Could you check a few things on this model? Use its own coordinates, in mm. A direction names the side the tool comes from. Round coordinates to 2 decimals unless told otherwise and drop trailing zeros. Order: outer loops, then holes, each group sorted by start corner. A loop starts at its lowest first (then second) coordinate and runs counter-clockwise, first axis right, second up. Notation, with made-up numbers: (50.5, 69) - (71.5, 69) arc R15 ccw to (71.5, 79) - close; hole circle Ø7 at (7.5, -31.5). An arc over 180 degrees is marked (long way). Use one line per item in the form item = value.
from build123d import *

# Parameters (mm, degrees)
F1_DEPTH = 63.5
F0_W     = 18.9613934278
F0_H     = 19.05
F2_DEPTH = 19.05
F3_DEPTH = 7.9375
F5_R     = 6.35


with BuildPart() as f1:
    # F0 (on Front) → F1 (new body, symmetric)
    with BuildSketch(Plane.XZ):
        Polygon((63.5, -19.05), (63.5, 19.05), (44.45, 19.05), (-63.5, 19.05), (-63.5, -19.05), align=None)
    extrude(amount=F1_DEPTH, both=True)

    # F0 (on Front) → F2 (join, symmetric)
    with BuildSketch(Plane.XZ):
        with Locations((98.3806967139, 73.025)):
            Rectangle(F0_W, F0_H)
        with BuildLine():
            Line((44.45, 19.05), (63.5, 19.05))
            Line((63.5, 19.05), (63.5, 50.8))
            ThreePointArc((63.5, 50.8), (67.2197438789, 59.7802561211), (76.2, 63.5))
            Line((76.2, 63.5), (88.9, 63.5))
            Line((88.9, 63.5), (88.9, 82.55))
            Line((88.9, 82.55), (76.2, 82.55))
            ThreePointArc((76.2, 82.55), (53.7493596973, 73.2506403027), (44.45, 50.8))
            Line((44.45, 50.8), (44.45, 19.05))
        make_face()
    extrude(amount=F2_DEPTH, both=True)

    # F0 (on Front) → F3 (join, symmetric)
    with BuildSketch(Plane.XZ):
        with BuildLine():
            Line((-63.5, 19.05), (44.45, 19.05))
            Line((44.45, 19.05), (44.45, 50.8))
            ThreePointArc((44.45, 50.8), (53.7493596973, 73.2506403027), (76.2, 82.55))
            add(Edge.make_bspline(
                [(-63.5, 19.05), (-43.5108728707, 70.1786652207), (14.7244036198, 83.1460282207), (76.2, 82.55)],
                knots=[0, 0, 0, 0, 153.4546838647, 153.4546838647, 153.4546838647, 153.4546838647], degree=3))
        make_face()
    extrude(amount=F3_DEPTH, both=True)

    # F0 (on Front) → F4 (revolve)
    with BuildSketch(Plane.XZ):
        Polygon((107.8613934278, 82.55), (107.8613934278, 63.5), (107.8613934278, 57.15), (127, 57.15), (127, 88.9), (107.8613934278, 88.9), align=None)
    revolve(axis=Axis((107.8613934278, 0, 73.025), (0, 0, 1)))

    # F5
    f5_edges = [f1.edges().sort_by_distance(p)[0] for p in [
        (-63.5, 63.5, 0),
        (-63.5, -63.5, 0),
        (63.5, -63.5, 0),
        (63.5, 63.5, 0),
    ]]
    fillet(f5_edges, radius=F5_R)


solid = f1.part
Item 1: Imagine slicing it at B-B on x = 97. Please give me the cut outline in (y, z), plus the area to 3 significant figures.
Found:
outline = (-19.05, 63.5) - (-15.76, 63.5) - (-15.76, 57.15) - (15.76, 57.15) - (15.76, 63.5) - (19.05, 63.5) - (19.05, 82.55) - (15.76, 82.55) - (15.76, 88.9) - (-15.76, 88.9) - (-15.76, 82.55) - (-19.05, 82.55) - close
area = 1,130 mm2
Item 2: Imagine slicing it at C-C on y = 52.5. Please give me the cut outline in (x, z).
Found:
outline = (-63.5, -19.05) - (63.5, -19.05) - (63.5, 19.05) - (-63.5, 19.05) - close
Item 3: Imagine slicing it at A-A on z = -4.5. Please give me the cut outline in (x, y), plus the area to 3 significant figures.
Found:
outline = (-63.5, -57.15) arc R6.35 ccw to (-57.15, -63.5) - (57.15, -63.5) arc R6.35 ccw to (63.5, -57.15) - (63.5, 57.15) arc R6.35 ccw to (57.15, 63.5) - (-57.15, 63.5) arc R6.35 ccw to (-63.5, 57.15) - close
area = 16,100 mm2
Item 4: I need wall thicknesses on L1, parallel to X at y = -12.5, z = 39; L2, parallel to Z at x = -30.5, y = 30.5; L3, parallel to Z at x = 119.5, y = -3. Which ranges of each line are inside material? Lowest first, please.
Found:
L1 = 44.45 to 63.5
L2 = -19.05 to 19.05
L3 = 57.15 to 88.9
Item 5: For faces 1 (the face through (63.5, -1, 8)), 2 (the face through (5, -7.938, 44)), which set-ups out of +Z, -Z, +X, -X, +Y, -Y let a thin tool reach every point of the face, with its end or its side?
Found:
face_1 = -Z, +X, +Y, -Y
face_2 = +Z, -X, -Y
Item 6: Will these pins go through, and if not, where does the flat tip stop? P1, Ø9, axis at y = 14.5, z = 38.5, coming from the -X side; P2, Ø1.5, axis at x = 35.5, z = 65.5, coming from the +Y side; P3, Ø1.5, axis at y = 30, z = 19.5, coming from the +X side.
Found:
P1 = 44.45
P2 = 7.94
P3 = 63.5
